Can you work these out from the model? Positions are in its coordinate system, mm. A direction names the side the tool comes from. Coordinates: 2 decimals unless noted, no trailing zeros. Order: outer loops, then holes, each group sorted by start corner. A loop starts at its lowest first (then second) coordinate and runs counter-clockwise, first axis right, second up. Notation, with made-up numbers: (-2.75, 70.5) -> (37.25, 70.5) arc R21 cw to (37.25, 94.5) -> close; hole circle Ø9 at (87, 68). An arc over 180 degrees is marked (long way). Write item = value, one per line.
```python
from build123d import *

# Parameters (mm, degrees)
BOSS_EXTRUDE1_DEPTH = 105
SKETCH3_R           = 2.75
CUT_EXTRUDE1_DEPTH  = 146.430395722
SKETCH5_R           = 1.5
CUT_EXTRUDE2_DEPTH  = 154.668474321
SKETCH7_W           = 24.871294837
SKETCH7_H           = 30
CUT_EXTRUDE5_DEPTH  = 19.5
FILLET1_R           = 19.5
CUT_EXTRUDE6_DEPTH  = 154.668474389
CUT_EXTRUDE8_DEPTH  = 146.430395795
FILLET2_R           = 10


with BuildPart() as part:
    # Sketch2 → Boss-Extrude1 (new body)
    with BuildSketch(Plane.XY):
        with BuildLine():
            Line((18.505, 30), (45, 30))
            Line((45, 30), (45, 90))
            Line((45, 90), (42, 90))
            Line((42, 90), (42, 33))
            Line((42, 33), (0, 33))
            Line((0, 33), (-25, 33))
            Line((-25, 33), (-25, 30))
            Line((-25, 30), (-5, 30))
            ThreePointArc((-5, 30), (-1.464466094, 28.535533906), (0, 25))
            Line((0, 25), (0, 0))
            Line((0, 0), (3, 0))
            Line((3, 0), (3, 30))
            Line((3, 30), (10.505, 30))
            Line((10.505, 30), (10.505, 0))
            Line((10.505, 0), (13.505, 0))
            Line((13.505, 0), (13.505, 25))
            ThreePointArc((13.505, 25), (14.969466094, 28.535533906), (18.505, 30))
        make_face()
    extrude(amount=BOSS_EXTRUDE1_DEPTH)

    # Sketch3 → Cut-Extrude1 (cut, through all)
    with BuildSketch(Plane.ZY):
        with Locations((26.25, 20.25)):
            Circle(SKETCH3_R)
        with Locations((78.75, 20.25)):
            Circle(SKETCH3_R)
    extrude(amount=-CUT_EXTRUDE1_DEPTH, mode=Mode.SUBTRACT)

    # Sketch5 → Cut-Extrude2 (cut, through all)
    with BuildSketch(Plane.ZY.offset(-42)):
        with Locations((4.9, 38.71)):
            Circle(SKETCH5_R)
        with Locations(Location((100.1, 38.71, 0), (0, 0, 180))):
            Circle(SKETCH5_R)
        with Locations((7.892916969, 82.187107172)):
            Circle(SKETCH5_R)
        with Locations(Location((97.107083031, 82.187107172, 0), (0, 0, 180))):
            Circle(SKETCH5_R)
    extrude(amount=-CUT_EXTRUDE2_DEPTH, mode=Mode.SUBTRACT)

    # Sketch7 → Cut-Extrude5 (cut)
    with BuildSketch(Plane(origin=(0, 0, 0), x_dir=(-1, 0, 0), z_dir=(0, 0, -1))):
        with Locations((-6.069352582, 15)):
            Rectangle(SKETCH7_W, SKETCH7_H)
    extrude(amount=-CUT_EXTRUDE5_DEPTH, mode=Mode.SUBTRACT)

    # Fillet1
    fillet1_edges = [part.edges().sort_by_distance(p)[0] for p in [
        (-1, 30, 19.5),
        (14.505, 30, 19.5),
    ]]
    fillet(fillet1_edges, radius=FILLET1_R - 0.0001)  # a hair under: the kernel refuses the full size

    # Sketch9 → Cut-Extrude6 (cut, through all)
    with BuildSketch(Plane.ZY.offset(-42)):
        with BuildLine():
            Line((23.4, 48.1), (81.6, 48.1))
            ThreePointArc((81.6, 48.1), (82.307106781, 47.807106781), (82.6, 47.1))
            Line((82.6, 47.1), (82.6, 41.1))
            ThreePointArc((82.6, 41.1), (82.307106781, 40.392893219), (81.6, 40.1))
            Line((81.6, 40.1), (23.4, 40.1))
            ThreePointArc((23.4, 40.1), (22.692893219, 40.392893219), (22.4, 41.1))
            Line((22.4, 41.1), (22.4, 47.1))
            ThreePointArc((22.4, 47.1), (22.692893219, 47.807106781), (23.4, 48.1))
        make_face()
    extrude(amount=-CUT_EXTRUDE6_DEPTH, mode=Mode.SUBTRACT)

    # Sketch10 → Cut-Extrude8 (cut, through all)
    with BuildSketch(Plane.ZY):
        Polygon((19.5, 0), (36.004964036, 0), (70.668478518, 0), (86.438146051, 0), (105, 0), (105, 9.649634618), (105, 25), (86.438146051, 25), (86.438146051, 9.649634618), (70.668478518, 9.649634618), (70.668478518, 25), (36.004964036, 25), (36.004964036, 9.649634618), (19.5, 9.649634618), align=None)
    extrude(amount=-CUT_EXTRUDE8_DEPTH, mode=Mode.SUBTRACT)

    # Fillet2
    fillet2_edges = [part.edges().sort_by_distance(p)[0] for p in [
        (1.5, 25, 36.004964036),
        (12.005, 25, 36.004964036),
        (1.5, 25, 70.668478518),
        (12.005, 25, 70.668478518),
        (1.5, 25, 86.438146051),
        (12.005, 25, 86.438146051),
    ]]
    fillet(fillet2_edges, radius=FILLET2_R)


solid = part.part
```
Item 1: I want a section at C-C, the plane y = 20.25. Give the number of separate pieces and of enclosed holes in the cut face, plus the area to 3 significant figures.
A:
separate_pieces = 8
enclosed_holes = 0
area = 170 mm2
Item 2: I want a section at A-A, the plane z = 26.25. Please give me the cut outline in (x, y) (3 decimals), plus the area to 3 significant figures.
A:
outline = (-25, 30) -> (-5, 30) arc R5 cw to (0, 25) -> (0, 23) -> (3, 23) -> (3, 30) -> (10.505, 30) -> (10.505, 23) -> (13.505, 23) -> (13.505, 25) arc R5 cw to (18.505, 30) -> (45, 30) -> (45, 40.1) -> (42, 40.1) -> (42, 33) -> (-25, 33) -> close; (0, 9.65) -> (3, 9.65) -> (3, 17.5) -> (0, 17.5) -> close; (10.505, 9.65) -> (13.505, 9.65) -> (13.505, 17.5) -> (10.505, 17.5) -> close; (42, 48.1) -> (45, 48.1) -> (45, 90) -> (42, 90) -> close
area = 457 mm2
Item 3: If we mould it in two halves opening along Y, with no side actions, what happens to faces 1 (the cylindrical face through (43.479, 37.246, 4.575)), 2 (the flat face through (1, 25, 53)), 3 (the flat face through (12, 12, 36.005))? For each: pulls with the +Y half, pulls with the -Y half, needs draft (parallel to the pull), parting line crosses it, or undercut.
A:
face_1 = undercut
face_2 = pulls with the -Y half
face_3 = needs draft
Item 4: For faces 4 (the flat face through (43, 40.1, 53)), 5 (the cylindrical face through (12.026, 22.148, 39.012)), 6 (the flat face through (44, 90, 52)), 7 (the flat face through (13.505, 17, 78)), 8 (the flat face through (9, 33, 52)), which set-ups out of +Z, -Z, +X, -X, +Y, -Y let a thin tool reach every point of the face, with its end or its side?
A:
face_4 = +X, -X
face_5 = +X, -X, -Y
face_6 = +Z, -Z, +X, -X, +Y
face_7 = +Z, -Z, +X, -Y
face_8 = +Z, -Z, -X, +Y
Item 5: If I drill on probe 1 along Y at (x, z) = (1.65, 26.25); probe 2 along Y at (x, z) = (1, 60.5); probe 3 along Y at (x, z) = (42.9, 100.1), over which ranges is the centre line in solid material (lowest first)?
A:
probe_1 = 9.65 to 17.5, 23 to 33
probe_2 = 25 to 33
probe_3 = 30 to 37.21, 40.21 to 90
Item 6: I want a section at D-D, the plane x = 21. Please give me the cut outline in (y, z).
A:
outline = (30, 0) -> (33, 0) -> (33, 105) -> (30, 105) -> close
Item 7: I want a section at B-B, the plane z = 58. Please give me the cut outline in (x, y) (3 decimals).
A:
outline = (-25, 30) -> (-5, 30) arc R5 cw to (0, 25) -> (3, 25) -> (3, 30) -> (10.505, 30) -> (10.505, 25) -> (13.505, 25) arc R5 cw to (18.505, 30) -> (45, 30) -> (45, 40.1) -> (42, 40.1) -> (42, 33) -> (-25, 33) -> close; (42, 48.1) -> (45, 48.1) -> (45, 90) -> (42, 90) -> close
Item 8: I'm going to push flat-ended pins straight in: P1, Ø12, axis at x = 6.5, z = 21.5, coming from the +Y side; P2, Ø2.5, axis at x = 12, y = 11, coming from the +Z side; P3, Ø4, axis at x = 17.5, z = 13.5, coming from the -Y side. Where does each tip first touch, or does it pass through?
A:
P1 = 33
P2 = 86.44
P3 = 29
